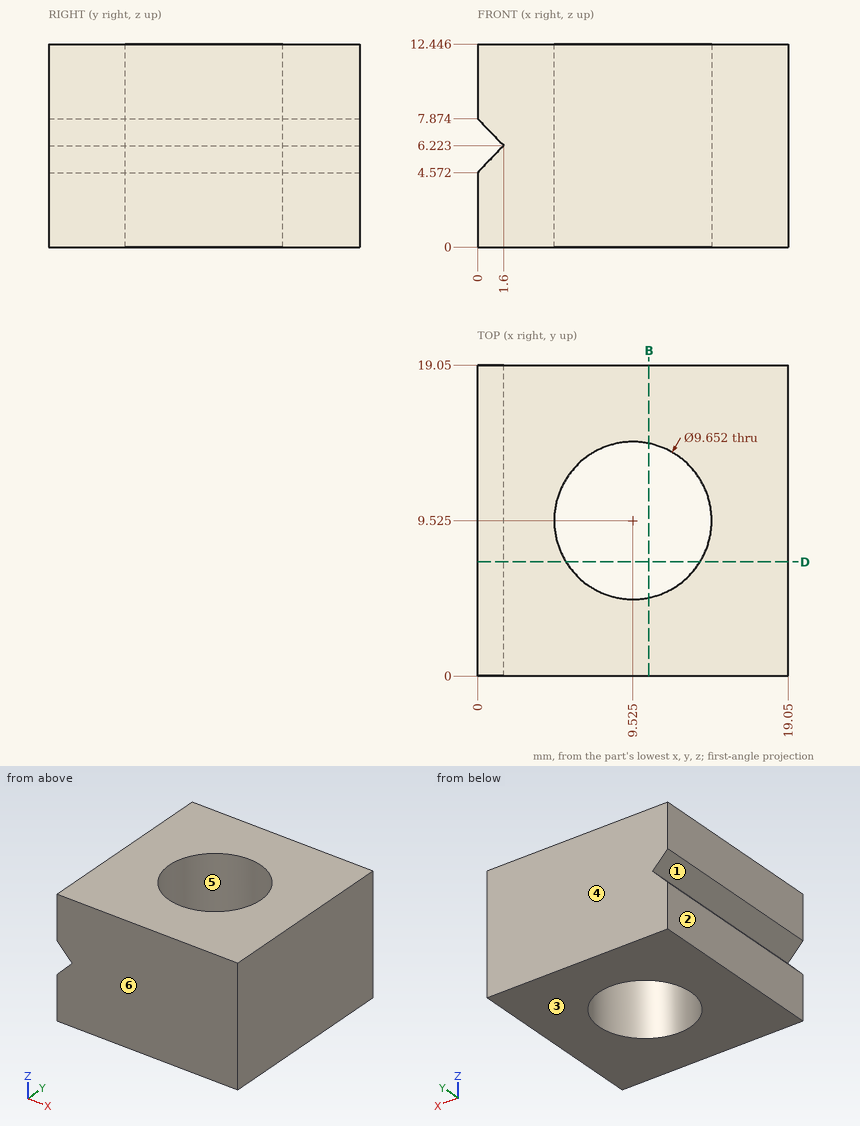
Here's the drawing with two shaded views (mm, measured from the low corner). I have some questions. A direction names the side the tool comes from. Give positions to 0.01 mm unless a question says otherwise; leave off trailing zeros. Write each loop counter-clockwise with the first axis right and the second up, starting at its lowest first coordinate (ties: lowest second). Pieces come first, ordered by that corner, then holes. Notation, with made-up numbers: (38.5, 52.5) -> (43.5, 52.5) arc R21 cw to (43.5, 56.5) -> close; hole circle Ø6 at (76.25, 12.5). An arc over 180 degrees is marked (long way). One line per item, written item: value.
Q1. We'd pull the mould along Y, two halves only. Please class the marked faces 3, 4, 5 and 6: +Y half, -Y half, draft (parallel to the pull), parting line (faces both ways), or undercut.
Results found:
face 3: draft
face 4: +Y half
face 5: undercut
face 6: -Y half
Q2. For P1, Ø8.5, axis at x = 9.525, y = 9.525, coming from the +Z side, with a flat end and sliding along its axis, tell me the tip position at first contact or that it passes through.
Results found:
P1: passes through
Q3. Which directions (+Z, -Z, +X, -X, +Y, -Y) give clear straight access to the entire face, cutting with the end or side of a thin tool? Please do the marked faces 1 and 2.
Results found:
face 1: -X, +Y, -Y
face 2: +Z, -Z, -X, +Y, -Y
Q4. Imagine slicing it at D-D on y = 7. Please give me the cut outline in (x, z).
Results found:
outline: (0, 0) -> (5.41, 0) -> (5.41, 12.45) -> (0, 12.45) -> (0, 7.87) -> (1.6, 6.22) -> (0, 4.57) -> close; (13.64, 0) -> (19.05, 0) -> (19.05, 12.45) -> (13.64, 12.45) -> close
Q5. Please list where these lines run through material, in increasing order: line 1 (X direction, y = 5.5, z = 1.5); line 2 (X direction, y = 6.25, z = 8); line 3 (Y direction, x = 10, z = 9). Write a range as [from, to].
Results found:
line 1: x = [0, 6.86], [12.19, 19.05]
line 2: x = [0, 5.98], [13.07, 19.05]
line 3: y = [0, 4.72], [14.33, 19.05]
Q6. Imagine slicing it at B-B on x = 10.5. Please give me the cut outline in (y, z), and give its area (3 significant figures).
Results found:
outline: (0, 0) -> (4.8, 0) -> (4.8, 12.45) -> (0, 12.45) -> close; (14.25, 0) -> (19.05, 0) -> (19.05, 12.45) -> (14.25, 12.45) -> close
area: 119 mm^2
